Autodesk Inventor part; units mm, degrees
ref_plane "YZ Plane" through (0, 0, 0) normal (1, 0, 0) x (0, 1, 0)
ref_plane "XZ Plane" through (0, 0, 0) normal (0, 1, 0) x (-1, 0, 0)
ref_plane "XY Plane" through (0, 0, 0) normal (0, 0, 1) x (1, 0, 0)
sketch "Sketch1" plane through (0, 0, 0) normal (0, 0, 1) x (1, 0, 0)
  line L0 (-16.5, -70) -> (16.5, -70)
  line L1 (16.5, -70) -> (16.5, 70)
  line L2 (16.5, 70) -> (-16.5, 70)
  line L3 (-16.5, 70) -> (-16.5, -70)
  line L4 (-16.5, -70) -> (16.5, 70) construction
  line L5 (16.5, -70) -> (-16.5, 70) construction
  line L6 (0, 70) -> (0, -70)
  line L7 (11.5, 30) -> (14.5, 30)
  line L8 (14.5, 30) -> (14.5, -30)
  line L9 (14.5, -30) -> (11.5, -30)
  line L10 (11.5, -30) -> (11.5, 30)
  circle A0 centre (0, 56) radius 5
  line L11 (-11.5, 30) -> (-14.5, 30)
  line L12 (-14.5, 30) -> (-14.5, -30)
  line L13 (-14.5, -30) -> (-11.5, -30)
  line L14 (-11.5, -30) -> (-11.5, 30)
  circle A1 centre (0, -60) radius 1.7
  circle A2 centre (-8.75, 36) radius 1.7
  circle A3 centre (8.75, 36) radius 1.7
  line L15 (-2.7129, 60.2) -> (2.7129, 60.2)
  point P0 (0, 0)
  point P1 (14.5, 0)
  point P2 (16.5, 0)
  point P3 (-14.5, 0)
  dimension "d1" = 140
  dimension "d2" = 3
  dimension "d3" = 2
  dimension "d4" = 60
  dimension "d5" = 10
  dimension "d6" = 14
  dimension "d7" = 3.4
  dimension "d8" = 10
  dimension "d9" = 3.4
  dimension "d10" = 23
  dimension "d11" = 20
  dimension "d21" = 4.2
  dimension "d22" = 17.5
sketch "Sketch3" plane through (0, 0, 1.5) normal (0, 0, 1) x (1, 0, 0)
  line L0 (-16.5, 70) -> (-16.5, -70)
  line L1 (-16.5, 70) -> (16.5, 70)
  line L2 (16.5, 70) -> (16.5, 90)
  line L3 (16.5, 90) -> (-16.5, 90)
  line L4 (-16.5, 90) -> (-16.5, 70)
  line L5 (16.5, 70) -> (16.5, -70)
  point P0 (0, 0)
  point P1 (16.5, 0)
  dimension "d24" = 20
extrude "Plate1" add sketch "Sketch1" along normal mid plane 3 contours L3 L2 L6 A0 A1 L0 | L6 A1 A0 L2 L1 L0 | A0 L15 L6 | L6 L15 A0 picked at (1.5261, 60.3463) picked at (-1.5261, 60.3463)
sheet face with bend "Face3" sketch "Sketch3" thickness 3 toward (0, 0, -1) bend radius 3
bend "Bend2"
equation "\"d13\" = Thickness"
equation "\"d25\" = BendRadius"
equation "\"d26\" = BendReliefWidth"
equation "\"d28\" = MinimumRemnant"
equation "\"d27\" = BendReliefDepth"
equation "\"d29\" = TransitionRadius"
equation "\"BendRadius\" = Thickness"
equation "\"BendReliefWidth\" = Thickness"
equation "\"BendReliefDepth\" = 0.5 * Thickness"
equation "\"CornerReliefSize\" = 4 * Thickness"
equation "\"MinimumRemnant\" = 2 * Thickness"
equation "\"TransitionRadius\" = BendRadius"
equation "\"JacobiRadiusSize\" = BendRadius"
equation "\"GapSize\" = Thickness"
properties part number "Motor Fixation .1"
Check sheet for the modelled part. Datum: model origin and axes. Units: mm. A direction names the side the tool comes from. Give positions to 0.01 mm unless a question says otherwise; leave off trailing zeros. Order: outer loops, then holes, each group sorted by start corner. A loop starts at its lowest first (then second) coordinate and runs counter-clockwise, first axis right, second up. Notation, with made-up numbers: (9, -35.75) - (52, -35.75) arc R14 cw to (52, -8.75) - close; hole circle Ø4 at (59.5, 81). An arc over 180 degrees is marked (long way). Answer as CSV lines item,"result".
1. Section check A-A (y = 56). Record the boundary of the cut face in (x, z), then the cut area to 3 significant figures.
Result sheet:
outline,"(-16.5, -1.5) - (-5, -1.5) - (-5, 1.5) - (-16.5, 1.5) - close; (5, -1.5) - (16.5, -1.5) - (16.5, 1.5) - (5, 1.5) - close"
area,"69.0 mm²"
2. Mould release check, pull along Y, two halves, no side actions. Record for faces 1 (the face through (16.5, 9, 0)), 2 (the face through (0, 90, 0)), 3 (the face through (-14.5, 0, 0)), 4 (the face through (0, 60.2, 0)): released by +Y, released by -Y, zero draft, split by the parting line, or undercut.
Result sheet:
face 1,"zero draft"
face 2,"released by +Y"
face 3,"undercut"
face 4,"undercut"
3. Section check D-D (z = -0.5). Record the boundary of the cut face in (x, y), then the cut area to 3 significant figures.
Result sheet:
outline,"(-16.5, -70) - (16.5, -70) - (16.5, 90) - (-16.5, 90) - close; hole (-14.5, -30) - (-11.5, -30) - (-11.5, 30) - (-14.5, 30) - close; hole circle Ø3.4 at (-8.75, 36); hole (-2.71, 60.2) arc R5 ccw (long way) to (2.71, 60.2) - close; hole circle Ø3.4 at (0, -60); hole circle Ø3.4 at (8.75, 36); hole (11.5, -30) - (14.5, -30) - (14.5, 30) - (11.5, 30) - close"
area,"4,820 mm²"
4. Section check C-C (y = -22). Record the boundary of the cut face in (x, z).
Result sheet:
outline,"(-16.5, -1.5) - (-14.5, -1.5) - (-14.5, 1.5) - (-16.5, 1.5) - close; (-11.5, -1.5) - (11.5, -1.5) - (11.5, 1.5) - (-11.5, 1.5) - close; (14.5, -1.5) - (16.5, -1.5) - (16.5, 1.5) - (14.5, 1.5) - close"
5. Tool access check on faces 5 (the face through (-11.5, 0, 0)), 6 (the face through (-16.5, 11, 0)). Record the directions out of +Z, -Z, +X, -X, +Y, -Y that give a thin tool (end or side, any length) a straight path to the whole face; none if there is none.
Result sheet:
face 5,"+Z, -Z"
face 6,"+Z, -Z, -X, +Y, -Y"
6. Section check B-B (x = 0). Record the boundary of the cut face in (y, z).
Result sheet:
outline,"(-70, -1.5) - (-61.7, -1.5) - (-61.7, 1.5) - (-70, 1.5) - close; (-58.3, -1.5) - (51, -1.5) - (51, 1.5) - (-58.3, 1.5) - close; (60.2, -1.5) - (90, -1.5) - (90, 1.5) - (60.2, 1.5) - close"
7. Scan lines: probe 1 along Y at (x, z) = (-8.75, 0.2); probe 2 along X at (y, z) = (56, -0.2); probe 3 along X at (y, z) = (28, 0.2). Record each from-to range of solid material in increasing order. Write a range as from..to.
Result sheet:
probe 1,"-70..34.3, 37.7..90"
probe 2,"-16.5..-5, 5..16.5"
probe 3,"-16.5..-14.5, -11.5..11.5, 14.5..16.5"
